```python
from build123d import *

# Parameters (mm, degrees)
SKETCH_1_R            = 40
EXTRUDE_1_DEPTH       = 20
SKETCH_2_R            = 22.5
CUT_EXTRUDE_1_DEPTH   = 61
CHAMFER_1_SIZE        = 1.5
SKETCH_3_R            = 2.5
CUT_EXTRUDE_597_DEPTH = 61
CHAMFER_2_SIZE        = 1


with BuildPart() as part:
    # Эскиз1 → Бобышка-Вытянуть1 (new body)
    with BuildSketch(Plane(origin=(0, 0, 0), x_dir=(1, 0, 0), z_dir=(0, 1, 0))):
        with Locations(Location((0, 0, 0), (0, 0, 270))):
            Circle(SKETCH_1_R)
    extrude(amount=EXTRUDE_1_DEPTH)

    # Эскиз2 → Вырез-Вытянуть1 (cut, through all)
    with BuildSketch(Plane(origin=(0, 20, 0), x_dir=(1, 0, 0), z_dir=(0, 1, 0))):
        with Locations(Location((0, 0, 0), (0, 0, 270))):
            Circle(SKETCH_2_R)
    extrude(amount=-CUT_EXTRUDE_1_DEPTH, mode=Mode.SUBTRACT)

    # Фаска1
    chamfer_1_edges = [part.edges().sort_by_distance(p)[0] for p in [
        (0, 0, -22.5),
        (0, 20, -22.5),
    ]]
    chamfer(chamfer_1_edges, length=CHAMFER_1_SIZE)

    # Эскиз3 → Cut-Extrude 597 (cut, through all)
    with BuildSketch(Plane.XZ):
        with Locations(Location((0, -30, 0), (0, 0, 270))):
            Circle(SKETCH_3_R)
    extrude(amount=-CUT_EXTRUDE_597_DEPTH, mode=Mode.SUBTRACT)

    # Фаска2
    chamfer_2_edges = [part.edges().sort_by_distance(p)[0] for p in [
        (0, 20, -27.5),
        (0, 0, -27.5),
    ]]
    chamfer(chamfer_2_edges, length=CHAMFER_2_SIZE)


solid = part.part
```
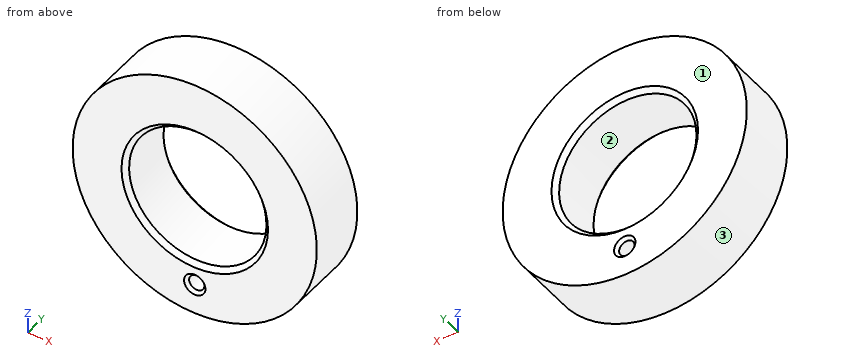
Can you work these out from the model? Positions are in its coordinate system, mm. Face numbers are marked on the shaded views. Give positions to 0.01 mm unless a question says otherwise; leave off trailing zeros. Loops run counter-clockwise (first coordinate to the right, second up) from the corner with the lowest first, then second, coordinate; pieces in that order, holes last. Notation, with made-up numbers: M 81,42.25 L 118,42.25 A21 cw 118,46.25 Z; hole C 61.5,72.25 d2. An arc over 180 degrees is marked long. Answer in a Markdown table with one row per item.
1. If I drill on line 1 along X through (y, z) = (10.5, 0); line 2 along Z through (x, y) = (2, 10.5); line 3 along Z through (x, y) = (20, 8.75), over which ranges is the centre line in solid material (lowest first)?
Taken from the geometry:
| item | result |
|---|---|
| line 1 | x = -40 to -22.5, 22.5 to 40 |
| line 2 | z = -39.95 to -31.5, -28.5 to -22.41, 22.41 to 39.95 |
| line 3 | z = -34.64 to -10.31, 10.31 to 34.64 |
2. Suppose I cut it at B-B on x = 0. Write out the boundary of the cut face in (y, z), plus the area to 4 significant figures.
Taken from the geometry:
| item | result |
|---|---|
| outline | M 0,-40 L 20,-40 L 20,-33.5 L 19,-32.5 L 1,-32.5 L 0,-33.5 Z; M 0,-26.5 L 1,-27.5 L 19,-27.5 L 20,-26.5 L 20,-24 L 18.5,-22.5 L 1.5,-22.5 L 0,-24 Z; M 0,24 L 1.5,22.5 L 18.5,22.5 L 20,24 L 20,40 L 0,40 Z |
| area | 593.5 mm² |
3. Suppose I cut it at C-C on y = 10. Write out the boundary of the cut face in (x, z).
Taken from the geometry:
| item | result |
|---|---|
| outline | C 0,0 d80; hole C 0,0 d45; hole C 0,-30 d5 |
4. Suppose I cut it at A-A on z = 0. Write out the boundary of the cut face in (x, y), plus the area to 4 significant figures.
Taken from the geometry:
| item | result |
|---|---|
| outline | M -40,0 L -24,0 L -22.5,1.5 L -22.5,18.5 L -24,20 L -40,20 Z; M 22.5,1.5 L 24,0 L 40,0 L 40,20 L 24,20 L 22.5,18.5 Z |
| area | 695.5 mm² |
5. Thinking about a two-plate mould opening in X: for the marked faces 1, 2 and 3, which applies, released by +X, released by -X, zero draft, split by the parting line, or undercut?
Taken from the geometry:
| item | result |
|---|---|
| face 1 | zero draft |
| face 2 | undercut |
| face 3 | split by the parting line |
6. Suppose I cut it at D-D on z = -30. Write out the boundary of the cut face in (x, y), plus the area to 3 significant figures.
Taken from the geometry:
| item | result |
|---|---|
| outline | M -26.46,0 L -3.5,0 L -2.5,1 L -2.5,19 L -3.5,20 L -26.46,20 Z; M 2.5,1 L 3.5,0 L 26.46,0 L 26.46,20 L 3.5,20 L 2.5,19 Z |
| area | 956 mm² |
7. For pin 1 Ø6 at (x, y) = (10.5, 10.5) entering from +Z; pin 2 Ø5 at (x, y) = (-15, 3) entering from +Z; pin 3 Ø6 at (y, z) = (15.5, 27.5) entering from +X, each with a flat end and sliding along its axis, tell me the tip position at first contact or that it passes through.
Taken from the geometry:
| item | result |
|---|---|
| pin 1 | stops at z = 39.29 |
| pin 2 | stops at z = 38 |
| pin 3 | stops at x = 31.62 |
